Design review of the part built by this model. Coordinates are the model's own, in mm. Round coordinates to 2 decimals unless told otherwise and drop trailing zeros. Order: outer loops, then holes, each group sorted by start corner. A loop starts at its lowest first (then second) coordinate and runs counter-clockwise, first axis right, second up. Notation, with made-up numbers: M 42,9 L 69,9 A23 ccw 69,32 Z; hole C 81,52.5 d10. An arc over 180 degrees is marked long. Use a Markdown table: item, result. Add a question column.
(1) Take a section at A-A (x = 0). Write out the cut boundary in (y, z).
(2) For pin 1 (4.5 mm diameter, centred on x = -1, z = -22.5, fed in from -Y); pin 2 (5.5 mm diameter, centred on x = 0, y = 0, fed in from -Z); pin 3 (3 mm diameter, centred on y = -1, z = 23, fed in from -X); pin 4 (2 mm diameter, centred on y = 2.5, z = -79.5, fed in from -X), all flat-tipped, find the tip position at first contact; note any pin that passes through.
(3) To check wall thickness, follow probe 1 along Y at (x, z) = (5, -47.5); probe 2 along Y at (x, z) = (7, 125); probe 3 along Y at (x, z) = (0, -90). State the ranges of each line that lie inside material, in increasing order. Write a range as from..to.
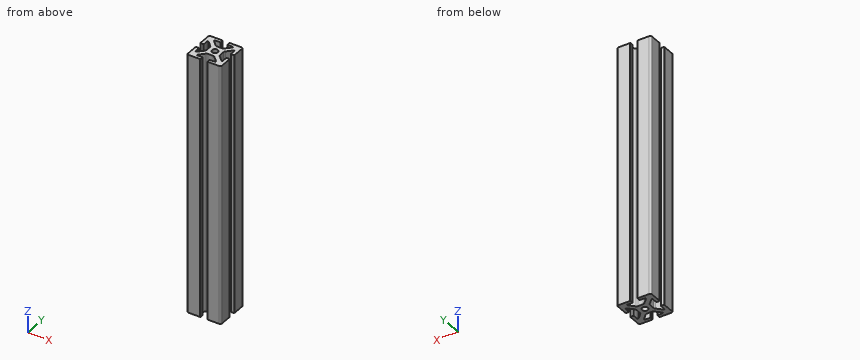
```python
from build123d import *

# Parameters (mm, degrees)
BOSS_EXTRUDE1_DEPTH      = 152.4
BOSS_EXTRUDE1_DEPTH_BACK = 152.4
SKETCH3_R                = 3.5


with BuildPart() as part:
    # Sketch3 → Boss-Extrude1 (new, two sides: drawn at the far end of the back side and taken through both)
    with BuildSketch(Plane.XY.offset(-BOSS_EXTRUDE1_DEPTH_BACK)):
        with BuildLine():
            Line((4.7874, 20), (18, 20))
            ThreePointArc((18, 20), (19.414213562, 19.414213562), (20, 18))
            Line((20, 18), (20, 4.7874))
            ThreePointArc((20, 4.7874), (19.76937588, 4.23062412), (19.2126, 4))
            Line((19.2126, 4), (16.3048, 4))
            ThreePointArc((16.3048, 4), (16.089273853, 4.089273853), (16, 4.3048))
            Line((16, 4.3048), (16, 10.1618))
            ThreePointArc((16, 10.1618), (15.482565253, 10.936195824), (14.569103096, 10.754496904))
            Line((14.569103096, 10.754496904), (8.878679656, 5.064073464))
            ThreePointArc((8.878679656, 5.064073464), (8.228361402, 4.090803418), (8, 2.942753121))
            Line((8, 2.942753121), (8, -2.942753121))
            ThreePointArc((8, -2.942753121), (8.228361402, -4.090803418), (8.878679656, -5.064073464))
            Line((8.878679656, -5.064073464), (14.569103096, -10.754496904))
            ThreePointArc((14.569103096, -10.754496904), (15.482565253, -10.936195824), (16, -10.1618))
            Line((16, -10.1618), (16, -4.3048))
            ThreePointArc((16, -4.3048), (16.089273853, -4.089273853), (16.3048, -4))
            Line((16.3048, -4), (19.2126, -4))
            ThreePointArc((19.2126, -4), (19.76937588, -4.23062412), (20, -4.7874))
            Line((20, -4.7874), (20, -18))
            ThreePointArc((20, -18), (19.414213562, -19.414213562), (18, -20))
            Line((18, -20), (4.7874, -20))
            ThreePointArc((4.7874, -20), (4.23062412, -19.76937588), (4, -19.2126))
            Line((4, -19.2126), (4, -16.3048))
            ThreePointArc((4, -16.3048), (4.089273853, -16.089273853), (4.3048, -16))
            Line((4.3048, -16), (10.1618, -16))
            ThreePointArc((10.1618, -16), (10.936195824, -15.482565253), (10.754496904, -14.569103096))
            Line((10.754496904, -14.569103096), (5.064073464, -8.878679656))
            ThreePointArc((5.064073464, -8.878679656), (4.090803418, -8.228361402), (2.942753121, -8))
            Line((2.942753121, -8), (-2.942753121, -8))
            ThreePointArc((-2.942753121, -8), (-4.090803418, -8.228361402), (-5.064073464, -8.878679656))
            Line((-5.064073464, -8.878679656), (-10.754496904, -14.569103096))
            ThreePointArc((-10.754496904, -14.569103096), (-10.936195824, -15.482565253), (-10.1618, -16))
            Line((-10.1618, -16), (-4.3048, -16))
            ThreePointArc((-4.3048, -16), (-4.089273853, -16.089273853), (-4, -16.3048))
            Line((-4, -16.3048), (-4, -19.2126))
            ThreePointArc((-4, -19.2126), (-4.23062412, -19.76937588), (-4.7874, -20))
            Line((-4.7874, -20), (-18, -20))
            ThreePointArc((-18, -20), (-19.414213562, -19.414213562), (-20, -18))
            Line((-20, -18), (-20, -4.7874))
            ThreePointArc((-20, -4.7874), (-19.76937588, -4.23062412), (-19.2126, -4))
            Line((-19.2126, -4), (-16.3048, -4))
            ThreePointArc((-16.3048, -4), (-16.089273853, -4.089273853), (-16, -4.3048))
            Line((-16, -4.3048), (-16, -10.1618))
            ThreePointArc((-16, -10.1618), (-15.482565253, -10.936195824), (-14.569103096, -10.754496904))
            Line((-14.569103096, -10.754496904), (-8.878679656, -5.064073464))
            ThreePointArc((-8.878679656, -5.064073464), (-8.228361402, -4.090803418), (-8, -2.942753121))
            Line((-8, -2.942753121), (-8, 2.942753121))
            ThreePointArc((-8, 2.942753121), (-8.228361402, 4.090803418), (-8.878679656, 5.064073464))
            Line((-8.878679656, 5.064073464), (-14.569103096, 10.754496904))
            ThreePointArc((-14.569103096, 10.754496904), (-15.482565253, 10.936195824), (-16, 10.1618))
            Line((-16, 10.1618), (-16, 4.3048))
            ThreePointArc((-16, 4.3048), (-16.089273853, 4.089273853), (-16.3048, 4))
            Line((-16.3048, 4), (-19.2126, 4))
            ThreePointArc((-19.2126, 4), (-19.76937588, 4.23062412), (-20, 4.7874))
            Line((-20, 4.7874), (-20, 18))
            ThreePointArc((-20, 18), (-19.414213562, 19.414213562), (-18, 20))
            Line((-18, 20), (-4.7874, 20))
            ThreePointArc((-4.7874, 20), (-4.23062412, 19.76937588), (-4, 19.2126))
            Line((-4, 19.2126), (-4, 16.3048))
            ThreePointArc((-4, 16.3048), (-4.089273853, 16.089273853), (-4.3048, 16))
            Line((-4.3048, 16), (-10.1618, 16))
            ThreePointArc((-10.1618, 16), (-10.936195824, 15.482565253), (-10.754496904, 14.569103096))
            Line((-10.754496904, 14.569103096), (-5.064073464, 8.878679656))
            ThreePointArc((-5.064073464, 8.878679656), (-4.090803418, 8.228361402), (-2.942753121, 8))
            Line((-2.942753121, 8), (2.942753121, 8))
            ThreePointArc((2.942753121, 8), (4.090803418, 8.228361402), (5.064073464, 8.878679656))
            Line((5.064073464, 8.878679656), (10.754496904, 14.569103096))
            ThreePointArc((10.754496904, 14.569103096), (10.936195824, 15.482565253), (10.1618, 16))
            Line((10.1618, 16), (4.3048, 16))
            ThreePointArc((4.3048, 16), (4.089273853, 16.089273853), (4, 16.3048))
            Line((4, 16.3048), (4, 19.2126))
            ThreePointArc((4, 19.2126), (4.23062412, 19.76937588), (4.7874, 20))
        make_face()
        with Locations(Location((0, 0, 0), (0, 0, 180))):
            Circle(SKETCH3_R, mode=Mode.SUBTRACT)
    extrude(amount=BOSS_EXTRUDE1_DEPTH + BOSS_EXTRUDE1_DEPTH_BACK)


solid = part.part
```
Verdict:
| question | item | result |
|---|---|---|
| 1 | outline | M -8,-152.4 L -3.5,-152.4 L -3.5,152.4 L -8,152.4 Z; M 3.5,-152.4 L 8,-152.4 L 8,152.4 L 3.5,152.4 Z |
| 2 | pin 1 | stops at y = -8.02 |
| 2 | pin 2 | passes through |
| 2 | pin 3 | stops at x = -8 |
| 2 | pin 4 | stops at x = -8.05 |
| 3 | probe 1 | y = -20..-16, -8.82..8.82, 16..20 |
| 3 | probe 2 | y = -20..-16, -10.81..10.81, 16..20 |
| 3 | probe 3 | y = -8..-3.5, 3.5..8 |
